Geometry check sheet. Reference: drawing and pictorial views, mm from the part's lowest x, y, z. A direction names the side the tool comes from. Coordinates: 2 decimals unless noted, no trailing zeros. Loops run counter-clockwise (first coordinate to the right, second up) from the corner with the lowest first, then second, coordinate; pieces in that order, holes last. Notation, with made-up numbers: (39.25, 34) -> (80.25, 34) arc R29 cw to (80.25, 63) -> close; hole circle Ø5 at (35, 83). An arc over 180 degrees is marked (long way). Use CSV: the item, a comma, the result in double quotes.
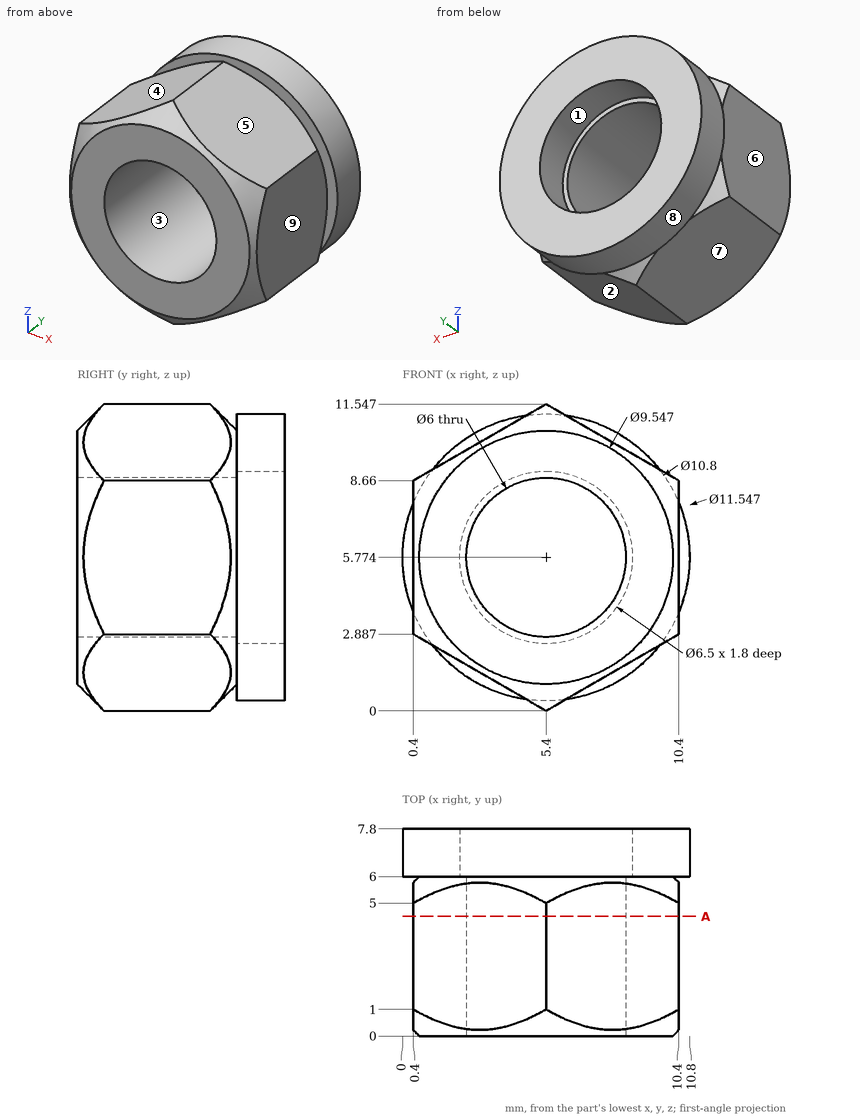
1) Thickness scan on line 1 along Z through (x, y) = (6, 0.5) (1 decimal); line 2 along Z through (x, y) = (6.75, 3) (1 decimal); line 3 along Y through (x, z) = (1, 3) (1 decimal). Record the ranges inside material, lowest first. Write a range as from..to.
Answer below:
line 1,"z = 0.5..2.8, 8.7..11"
line 2,"z = 0.8..3.1, 8.5..10.8"
line 3,"y = 0.4..5.6, 6..7.8"
2) Draft check along X on the marked faces 1, 2, 3 and 4. Enter one of: released by +X, released by -X, zero draft, split by the parting line, or undercut.
Answer below:
face 1,"undercut"
face 2,"released by +X"
face 3,"undercut"
face 4,"released by -X"
3) Cross-section at A-A on y = 4.5. Record the boundary of the cut face in (x, z).
Answer below:
outline,"(0.4, 2.89) -> (5.4, 0) -> (10.4, 2.89) -> (10.4, 8.66) -> (5.4, 11.55) -> (0.4, 8.66) -> close; hole circle Ø6 at (5.4, 5.77)"
4) Access from +Z, -Z, +X, -X, +Y, -Y to the whole of each face (thin tool, end or side, straight path). Record for the marked faces 5, 6, 7, 8 and 9.
Answer below:
face 5,"+Z, +X, -Y"
face 6,"+Z, -Z, -X, -Y"
face 7,"-Z, -X, -Y"
face 8,"+Y"
face 9,"+Z, -Z, +X, -Y"
5) Go/stop test with flat-tipped pins: pin 1 Ø2 at (y, z) = (3, 8) entering from -X; pin 2 Ø3 at (y, z) = (4, 4.5) entering from +X; pin 3 Ø4.5 at (y, z) = (4, 7) entering from -X. Record where each tip stops, or that it passes through.
Answer below:
pin 1,"stops at x = 0.4"
pin 2,"stops at x = 10.4"
pin 3,"stops at x = 0"
